from build123d import *

# Parameters (mm, degrees)
SKETCH_R                   = 1.62
EXTRUDE_SKETCH_DEPTH       = 1.5
RECTANGLE004_W             = 20.8
RECTANGLE004_H             = 2.4
EXTRUDE_RECTANGLE004_DEPTH = 9
EXTRUDE_SKETCH002_DEPTH    = 1
SKETCH001_W                = 35
SKETCH001_H                = 7
EXTRUDE_SKETCH001_DEPTH    = 3
CHAMFER_SIZE               = 0.5
RECTANGLE006_W             = 35.4
RECTANGLE006_H             = 10
EXTRUDE_RECTANGLE006_DEPTH = 5
RECTANGLE001_W             = 15.6
RECTANGLE001_H             = 2.4
EXTRUDE_RECTANGLE001_DEPTH = 9
RECTANGLE_W                = 20.7
RECTANGLE_H                = 2.4
EXTRUDE_RECTANGLE_DEPTH    = 9
RECTANGLE009_W             = 9
RECTANGLE009_H             = 11
EXTRUDE_RECTANGLE009_DEPTH = 3
EXTRUDE_SKETCH005_DEPTH    = 11
RECTANGLE008_W             = 16
RECTANGLE008_H             = 12
EXTRUDE_RECTANGLE008_DEPTH = 11.7
SKETCH003_W                = 6
SKETCH003_H                = 6
EXTRUDE_SKETCH003_DEPTH    = 2
SKETCH004_R                = 1.5
EXTRUDE_SKETCH004_DEPTH    = 1.5
RECTANGLE003_W             = 25.8
RECTANGLE003_H             = 2.4
EXTRUDE_RECTANGLE003_DEPTH = 9


with BuildPart() as sketch_extrude:
    # Sketch → Extrude_Sketch (new body)
    with BuildSketch(Plane.XY):
        with BuildLine():
            Line((1, 0), (65.4, 0))
            ThreePointArc((65.4, 0), (66.107107, 0.292893), (66.4, 1))
            Line((66.4, 1), (66.4, 2.55))
            Line((68.95, 5.1), (66.4, 2.55))
            Line((68.95, 38.05), (68.95, 5.1))
            Line((66.4, 40.6), (68.95, 38.05))
            Line((66.4, 40.6), (66.4, 52.1))
            Line((64.85, 53.65), (66.4, 52.1))
            Line((64.85, 53.65), (1, 53.65))
            ThreePointArc((1, 53.65), (0.292893, 53.357107), (0, 52.65))
            Line((0, 52.65), (0, 1))
            ThreePointArc((0, 1), (0.292893, 0.292893), (1, 0))
        make_face()
        with Locations((14.05247, 2.556984)):
            Circle(SKETCH_R, mode=Mode.SUBTRACT)
        with Locations((15.334135, 51.082933)):
            Circle(SKETCH_R, mode=Mode.SUBTRACT)
        with Locations((66.409951, 35.749834)):
            Circle(SKETCH_R, mode=Mode.SUBTRACT)
        with Locations((66.413926, 7.668398)):
            Circle(SKETCH_R, mode=Mode.SUBTRACT)
    extrude(amount=EXTRUDE_SKETCH_DEPTH)


with BuildPart() as rectangle004_extrude:
    # Rectangle004 (on Extrude_Sketch) → Extrude_Rectangle004 (new body)
    with BuildSketch(Plane(origin=(44.6, 49.85, 1.5), x_dir=(1, 0, 0), z_dir=(0, 0, 1))):
        with Locations((10.4, 1.2)):
            Rectangle(RECTANGLE004_W, RECTANGLE004_H)
    extrude(amount=EXTRUDE_RECTANGLE004_DEPTH)


with BuildPart() as sketch002_extrude:
    # Sketch002 (on Face6 of Extrude_Sketch001) → Extrude_Sketch002 (new body)
    with BuildSketch(Plane.XY.offset(9.5)):
        with BuildLine():
            Line((29, 13), (64, 13))
            Line((64, 13), (64, 15.5))
            ThreePointArc((64, 17.5), (63, 16.5), (64, 15.5))
            Line((64, 17.5), (64, 20))
            Line((64, 20), (29, 20))
            Line((29, 20), (29, 13))
        make_face()
    extrude(amount=EXTRUDE_SKETCH002_DEPTH)


with BuildPart() as chamfer_body:
    # Sketch001 (on Face6 of Extrude_Rectangle006) → Extrude_Sketch001 (new body)
    with BuildSketch(Plane.XY.offset(6.5)):
        with Locations((46.5, 16.5)):
            Rectangle(SKETCH001_W, SKETCH001_H)
    extrude(amount=EXTRUDE_SKETCH001_DEPTH)

    # Fusion: union Sketch002_Extrude
    add(sketch002_extrude.part)

    # Chamfer
    chamfer_edges = [chamfer_body.edges().sort_by_distance(p)[0] for p in [
        (46.5, 13, 10.5),
        (46.5, 20, 10.5),
    ]]
    chamfer(chamfer_edges, length=CHAMFER_SIZE)


with BuildPart() as rectangle006_extrude:
    # Rectangle006 (on Extrude_Sketch) → Extrude_Rectangle006 (new body)
    with BuildSketch(Plane(origin=(29, 11.5, 1.5), x_dir=(1, 0, 0), z_dir=(0, 0, 1))):
        with Locations((17.7, 5)):
            Rectangle(RECTANGLE006_W, RECTANGLE006_H)
    extrude(amount=EXTRUDE_RECTANGLE006_DEPTH)


with BuildPart() as rectangle001_extrude:
    # Rectangle001 (on Extrude_Sketch) → Extrude_Rectangle001 (new body)
    with BuildSketch(Plane(origin=(49.2, 1.4, 1.5), x_dir=(1, 0, 0), z_dir=(0, 0, 1))):
        with Locations((7.8, 1.2)):
            Rectangle(RECTANGLE001_W, RECTANGLE001_H)
    extrude(amount=EXTRUDE_RECTANGLE001_DEPTH)


with BuildPart() as rectangle_extrude:
    # Rectangle (on Extrude_Sketch) → Extrude_Rectangle (new body)
    with BuildSketch(Plane(origin=(26.6, 1.4, 1.5), x_dir=(1, 0, 0), z_dir=(0, 0, 1))):
        with Locations((10.35, 1.2)):
            Rectangle(RECTANGLE_W, RECTANGLE_H)
    extrude(amount=EXTRUDE_RECTANGLE_DEPTH)


with BuildPart() as rectangle009_extrude:
    # Rectangle009 (on Extrude_Sketch) → Extrude_Rectangle009 (new body)
    with BuildSketch(Plane(origin=(-1.5, 13.5, 1.5), x_dir=(0, -1, 0), z_dir=(-1, 0, 0))):
        with Locations((4.5, 5.5)):
            Rectangle(RECTANGLE009_W, RECTANGLE009_H)
    extrude(amount=-EXTRUDE_RECTANGLE009_DEPTH)


with BuildPart() as fusion001:
    # Sketch005 (on Face6 of Extrude_Rectangle009) → Extrude_Sketch005 (new body)
    with BuildSketch(Plane.YZ.offset(1.5)):
        with BuildLine():
            Line((4.5, 1.5), (13.5, 1.5))
            Line((13.5, 1.5), (13.5, 7.5))
            Line((13.5, 7.5), (13, 7.5))
            ThreePointArc((13, 7.5), (9, 11.5), (5, 7.5))
            Line((5, 7.5), (4.5, 7.5))
            Line((4.5, 7.5), (4.5, 1.5))
        make_face()
    extrude(amount=EXTRUDE_SKETCH005_DEPTH)

    # Fusion001: union Rectangle009_Extrude
    add(rectangle009_extrude.part)


with BuildPart() as rectangle008_extrude:
    # Rectangle008 → Extrude_Rectangle008 (new body)
    with BuildSketch(Plane(origin=(-6.4, 32, 1.5), x_dir=(1, 0, 0), z_dir=(0, 0, 1))):
        with Locations((8, 6)):
            Rectangle(RECTANGLE008_W, RECTANGLE008_H)
    extrude(amount=EXTRUDE_RECTANGLE008_DEPTH)


with BuildPart() as sketch003_extrude:
    # Sketch003 (on Face18 of Extrude_Sketch) → Extrude_Sketch003 (new body)
    with BuildSketch(Plane.XY.offset(1.5)):
        with Locations((6, 50)):
            Rectangle(SKETCH003_W, SKETCH003_H)
    extrude(amount=EXTRUDE_SKETCH003_DEPTH)


with BuildPart() as sketch004_extrude:
    # Sketch004 (on Face6 of Extrude_Sketch003) → Extrude_Sketch004 (new body)
    with BuildSketch(Plane.XY.offset(3.5)):
        with Locations((6, 50)):
            Circle(SKETCH004_R)
    extrude(amount=EXTRUDE_SKETCH004_DEPTH)


with BuildPart() as arduino:
    # Rectangle003 (on Extrude_Sketch) → Extrude_Rectangle003 (new body)
    with BuildSketch(Plane(origin=(18, 49.85, 1.5), x_dir=(1, 0, 0), z_dir=(0, 0, 1))):
        with Locations((12.9, 1.2)):
            Rectangle(RECTANGLE003_W, RECTANGLE003_H)
    extrude(amount=EXTRUDE_RECTANGLE003_DEPTH)

    # Fusion002: union Rectangle004_Extrude, Chamfer body, Rectangle006_Extrude, Rectangle001_Extrude, Rectangle_Extrude, Fusion001, Rectangle008_Extrude, Sketch003_Extrude, Sketch004_Extrude
    add(rectangle004_extrude.part)
    add(chamfer_body.part)
    add(rectangle006_extrude.part)
    add(rectangle001_extrude.part)
    add(rectangle_extrude.part)
    add(fusion001.part)
    add(rectangle008_extrude.part)
    add(sketch003_extrude.part)
    add(sketch004_extrude.part)

    # Fusion003: union Sketch_Extrude
    add(sketch_extrude.part)


with BuildPart() as arduino_1:
    # Fusion003 placement: moved
    add(arduino.part.moved(Location((1, 1, 3))))


solid = arduino_1.part
Part model, mm, in its own coordinate system. A direction names the side the tool comes from. Give positions to 0.01 mm unless a question says otherwise; leave off trailing zeros. Write each loop counter-clockwise with the first axis right and the second up, starting at its lowest first coordinate (ties: lowest second). Pieces come first, ordered by that corner, then holes.
1) Pin check, flat tips, straight feed: pin 1 (4.5 mm diameter, centred on x = 32.5, z = 8, fed in from +Y); pin 2 (1.2 mm diameter, centred on y = 4, z = 11, fed in from -X); pin 3 (3 mm diameter, centred on x = 55.5, y = 17, fed in from +Z); pin 4 (1.9 mm diameter, centred on x = 16.33, y = 52.08, fed in from +Z). Stop position of each tip, or through.
Resolved:
pin 1: stops at y = 53.25
pin 2: stops at x = 27.6
pin 3: stops at z = 13.5
pin 4: passes through
2) Cut at A-A on x = 21. Write the cut outline in (y, z).
Resolved:
outline: (1, 3) - (54.65, 3) - (54.65, 4.5) - (53.25, 4.5) - (53.25, 13.5) - (50.85, 13.5) - (50.85, 4.5) - (1, 4.5) - close
3) Probe L1, parallel to Y at x = 56, z = 9.25; L2, parallel to Y at x = 56, z = 10.5; L3, parallel to Y at x = 8, z = 8.5. List the from-to ranges inside material, lowest first.
Resolved:
L1: y = 2.4 to 4.8, 12.5 to 22.5, 50.85 to 53.25
L2: y = 2.4 to 4.8, 14 to 21, 50.85 to 53.25
L3: y = 5.5 to 14.5, 33 to 45
4) Cut at B-B on y = 19.5. Write the cut outline in (x, z), then the cut area to 3 significant figures.
Resolved:
outline: (1, 3) - (69.95, 3) - (69.95, 4.5) - (65.4, 4.5) - (65.4, 9.5) - (65, 9.5) - (65, 13.5) - (30, 13.5) - (30, 4.5) - (1, 4.5) - close
area: 420 mm2
5) Which spindle directions (+Z, -Z, +X, -X, +Y, -Y) get a long thin tool onto all of the face, cutting with end or side? Do faces 1 (the face through (4, 51, 5)), 2 (the face through (7, 48, 5)), 3 (the face through (5.6, 52.4, 6.5)), 4 (the face through (50.2, 4, 9)). Say none if no direction does.
Resolved:
face 1: +Z, -X, +Y
face 2: +Z, +X, -X
face 3: +Z
face 4: +Z, -Y
6) Two-plate mould, pull along Y, no slides. Class faces 5 (the face through (58, 2.4, 9)), 6 (the face through (44.8, 52, 9)), 7 (the face through (56, 50.85, 9)): released by +Y, released by -Y, zero draft, split by the parting line, or undercut.
Resolved:
face 5: released by -Y
face 6: zero draft
face 7: undercut
7) Cut at C-C on x = 55. Write the cut outline in (y, z), then the cut area to 3 significant figures.
Resolved:
outline: (1, 3) - (54.65, 3) - (54.65, 4.5) - (53.25, 4.5) - (53.25, 13.5) - (50.85, 13.5) - (50.85, 4.5) - (22.5, 4.5) - (22.5, 9.5) - (21, 9.5) - (21, 13) - (20.5, 13.5) - (14.5, 13.5) - (14, 13) - (14, 9.5) - (12.5, 9.5) - (12.5, 4.5) - (4.8, 4.5) - (4.8, 13.5) - (2.4, 13.5) - (2.4, 4.5) - (1, 4.5) - close
area: 201 mm2
